Drawing for the job (mm, zero at the part's lowest x, y, z). A direction names the side the tool comes from. Round coordinates to 2 decimals unless told otherwise and drop trailing zeros. Order: outer loops, then holes, each group sorted by start corner. A loop starts at its lowest first (then second) coordinate and runs counter-clockwise, first axis right, second up. Notation, with made-up numbers: (86, 34.25) - (116, 34.25) arc R14 ccw to (116, 49.25) - close; hole circle Ø5 at (13.5, -5). An arc over 180 degrees is marked (long way). Put each result on its own line as item: value. Start each with the question number.
Item 1: Saw through at D-D on z = 145. List the corners of the cut face in (x, y), plus the area to 3 significant figures.
Item 2: Pin check, flat tips, straight feed: pin 1 Ø1 at (y, z) = (12, 27) entering from +X; pin 2 Ø10 at (y, z) = (28, 73) entering from -X; pin 3 Ø10 at (y, z) = (23, 106.5) entering from +X. Stop position of each tip, or through.
Item 3: Saw through at C-C on z = 126. List the corners of the cut face in (x, y), plus the area to 3 significant figures.
Item 4: Which spindle directions (+Z, -Z, +X, -X, +Y, -Y) get a long thin tool onto all of the face, cutting with end or side? Do the marked faces 1 and 2. Say none if no direction does.
Item 5: Probe probe 1 along Y at (x, z) = (16.5, 145); probe 2 along Z at (x, y) = (25, 9.5); probe 3 along Z at (x, y) = (30, 14). List the from-to ranges inside material, lowest first.
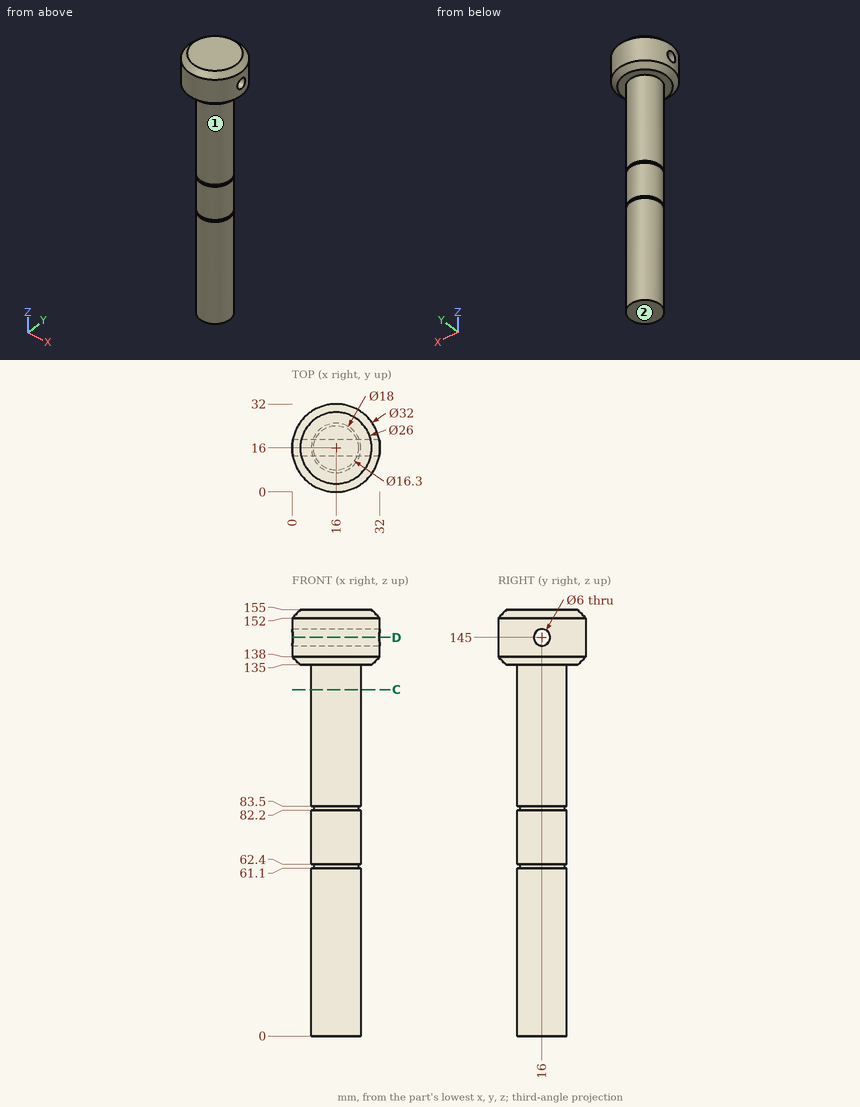
Results found:
1. outline: (0.28, 13) arc R16 ccw to (31.72, 13) - close; (0.28, 19) - (31.72, 19) arc R16 ccw to start
1. area: 613 mm²
2. pin 1: stops at x = 24.29
2. pin 2: stops at x = 10.34
2. pin 3: stops at x = 24.77
3. outline: circle Ø18 at (16, 16)
3. area: 254 mm²
4. face 1: -Z
4. face 2: -Z, +X, -X, +Y, -Y
5. probe 1: y = 0.01 to 13, 19 to 31.99
5. probe 2: z = 135 to 155
5. probe 3: z = 136.14 to 142.76, 147.24 to 153.86
